```python
from build123d import *

# Parameters (mm, degrees)
F0_R     = 19.05
F1_DEPTH = 50.8
F2_DEPTH = 50.8
F3_DEPTH = 50.8


with BuildPart() as f1:
    # F0 (on Front) → F1 (new body, symmetric)
    with BuildSketch(Plane.XZ):
        Circle(F0_R)
    extrude(amount=F1_DEPTH, both=True)

    # F2 (add): a face of the model
    f2_faces = [f1.faces().sort_by_distance(p)[0] for p in [
        (0, -50.8, 0),
    ]]
    extrude(f2_faces, amount=F2_DEPTH)

    # F3 (add): a face of the model
    f3_faces = [f1.faces().sort_by_distance(p)[0] for p in [
        (0, 50.8, 0),
    ]]
    extrude(f3_faces, amount=F3_DEPTH)


solid = f1.part
```
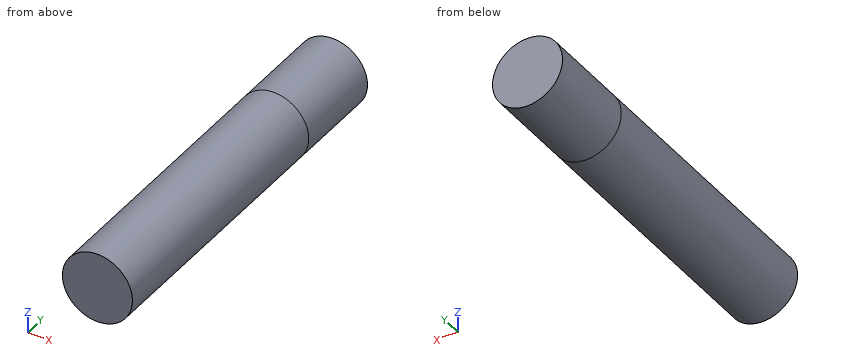
Geometry check sheet. Reference: the model listing, model coordinates, mm. Give positions to 0.01 mm unless a question says otherwise; leave off trailing zeros. Loops run counter-clockwise (first coordinate to the right, second up) from the corner with the lowest first, then second, coordinate; pieces in that order, holes last. Notation, with made-up numbers: M 70,6.25 L 79,6.25 A14 ccw 79,23.25 Z; hole C 22,43.25 d8. An arc over 180 degrees is marked long. Answer as CSV lines item,"result".
Item 1: Cross-section at C-C on x = -7.5. Record the cut outline in (y, z).
Values:
outline,"M -101.6,-17.51 L 101.6,-17.51 L 101.6,17.51 L -101.6,17.51 Z"
Item 2: Material ranges on line 1 (Z direction, x = 1, y = -80); line 2 (Z direction, x = -7, y = 61); line 3 (X direction, y = 37, z = 0.5), recorded low to high.
Values:
line 1,"z = -19.02 to 19.02"
line 2,"z = -17.72 to 17.72"
line 3,"x = -19.04 to 19.04"
Item 3: Cross-section at B-B on z = 11. Record the cut outline in (x, y), and give its area (3 significant figures).
Values:
outline,"M -15.55,-101.6 L 15.55,-101.6 L 15.55,101.6 L -15.55,101.6 Z"
area,"6,320 mm²"
Item 4: Depth check by flat-ended pin: P1, Ø1.5, axis at y = 5.5, z = -7, coming from the +X side; P2, Ø1.5, axis at x = -2, y = 73, coming from the -Z side; P3, Ø8, axis at x = -14, y = -41.5, coming from the +Z side; P4, Ø4, axis at y = -32, z = -1, coming from the +X side. Enter the tip coordinate at first touch or a pass-through.
Values:
P1,"stops at x = 18"
P2,"stops at z = -19.01"
P3,"stops at z = 16.21"
P4,"stops at x = 19.05"
Item 5: Cross-section at A-A on y = 81.5. Record the cut outline in (x, z), and give its area (3 significant figures).
Values:
outline,"C 0,0 d38.1"
area,"1,140 mm²"
